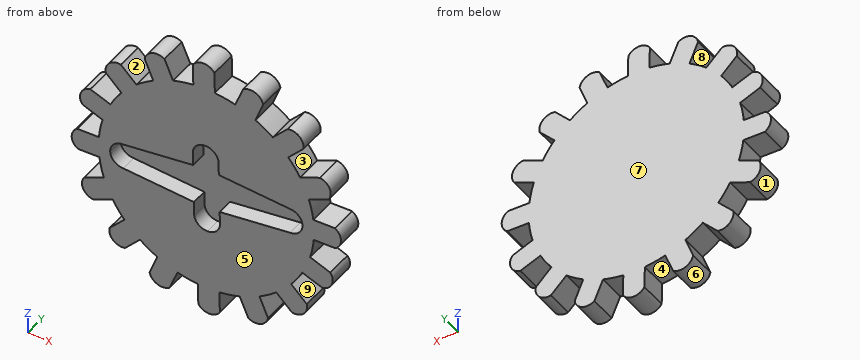
```python
from build123d import *

# Parameters (mm, degrees)
EXTRUDE001_DEPTH                      = 3
EXTRUDE001_ONTO_SKETCH001_ROLL_ANGLE  = -90
EXTRUDE001_ONTO_SKETCH001_PITCH_ANGLE = -1.786809
EXTRUDE_DEPTH                         = 5
EXTRUDE_ONTO_SKETCH_ROLL_ANGLE        = -90
EXTRUDE_ONTO_SKETCH_PITCH_ANGLE       = -1.786809
CUT_PITCH_ANGLE                       = 3
CUT_PLACEMENT_ANGLE                   = 180


with BuildPart() as servo_horn_gap:
    # Sketch001 as drawn → Extrude001 (new)
    with BuildSketch(Plane.XY):
        with BuildLine():
            Line((-2.39133, 6.362213), (-2.39133, 3.691866))
            Line((-2.39133, 3.691866), (-15.4752, 2.398726))
            ThreePointArc((-15.4752, 2.398726), (-17.158439, 1.689111), (-17.85396, 0))
            ThreePointArc((-17.85396, 0), (-17.158439, -1.689111), (-15.4752, -2.398726))
            Line((-2.39133, -3.691866), (-15.4752, -2.398726))
            Line((-2.39133, -6.362213), (-2.39133, -3.691866))
            ThreePointArc((-2.39133, -6.362213), (-1.613755, -7.907248), (0, -8.529784))
            ThreePointArc((0, -8.529784), (1.613755, -7.907248), (2.39133, -6.362213))
            Line((2.39133, -6.362213), (2.39133, -3.691866))
            Line((2.39133, -3.691866), (15.4752, -2.398726))
            ThreePointArc((15.4752, -2.398726), (17.158439, -1.689111), (17.85396, 0))
            ThreePointArc((17.85396, 0), (17.158439, 1.689111), (15.4752, 2.398726))
            Line((2.39133, 3.691866), (15.4752, 2.398726))
            Line((2.39133, 6.362213), (2.39133, 3.691866))
            ThreePointArc((2.39133, 6.362213), (1.613755, 7.907248), (0, 8.529784))
            ThreePointArc((0, 8.529784), (-1.613755, 7.907248), (-2.39133, 6.362213))
        make_face()
    extrude(amount=EXTRUDE001_DEPTH)


with BuildPart() as servo_horn_gap_1:
    # Extrude001 onto Sketch001 roll: moved
    add(servo_horn_gap.part.rotate(Axis((0, 0, 0), (1, 0, 0)), EXTRUDE001_ONTO_SKETCH001_ROLL_ANGLE))


with BuildPart() as servo_horn_gap_2:
    # Extrude001 onto Sketch001 pitch: moved
    add(servo_horn_gap_1.part.rotate(Axis((0, 0, 0), (0, 1, 0)), EXTRUDE001_ONTO_SKETCH001_PITCH_ANGLE))


with BuildPart() as servo_horn_gap_3:
    # Extrude001 onto Sketch001 placement: moved
    add(servo_horn_gap_2.part.moved(Location((16.5, 34.45, -6.25))))


with BuildPart() as servo_gear_mount:
    # Sketch as drawn → Extrude (new)
    with BuildSketch(Plane.XY):
        with BuildLine():
            ThreePointArc((-5.767545, -19.150337), (-3.901806, -19.615706), (-2, -19.899749))
            Line((-2, -19.899749), (-2, -23.899749))
            ThreePointArc((-2, -23.899749), (0, -25), (2, -23.899749))
            Line((2, -19.899749), (2, -23.899749))
            ThreePointArc((2, -19.899749), (3.901806, -19.615706), (5.767545, -19.150337))
            Line((5.767545, -19.150337), (7.298279, -22.845856))
            ThreePointArc((7.298279, -22.845856), (9.568651, -23.096339), (10.994375, -21.311783))
            Line((9.487389, -17.606518), (10.994375, -21.311783))
            ThreePointArc((9.487389, -17.606518), (11.122885, -16.621715), (12.657034, -15.485461))
            Line((12.657034, -15.485461), (15.485461, -18.313888))
            ThreePointArc((15.485461, -18.313888), (17.67767, -17.67767), (18.313888, -15.485461))
            Line((15.485461, -12.657034), (18.313888, -15.485461))
            ThreePointArc((15.485461, -12.657034), (16.621715, -11.122885), (17.606518, -9.487389))
            Line((17.606518, -9.487389), (21.311783, -10.994375))
            ThreePointArc((21.311783, -10.994375), (23.096339, -9.568651), (22.845856, -7.298279))
            Line((19.150337, -5.767545), (22.845856, -7.298279))
            ThreePointArc((19.150337, -5.767545), (19.615706, -3.901806), (19.899749, -2))
            Line((19.899749, -2), (23.899749, -2))
            ThreePointArc((23.899749, -2), (25, 0), (23.899749, 2))
            Line((19.899749, 2), (23.899749, 2))
            ThreePointArc((19.899749, 2), (19.615706, 3.901806), (19.150337, 5.767545))
            Line((19.150337, 5.767545), (22.845856, 7.298279))
            ThreePointArc((22.845856, 7.298279), (23.096339, 9.568651), (21.311783, 10.994375))
            Line((17.606518, 9.487389), (21.311783, 10.994375))
            ThreePointArc((17.606518, 9.487389), (16.621715, 11.122885), (15.485461, 12.657034))
            Line((15.485461, 12.657034), (18.313888, 15.485461))
            ThreePointArc((18.313888, 15.485461), (17.67767, 17.67767), (15.485461, 18.313888))
            Line((12.657034, 15.485461), (15.485461, 18.313888))
            ThreePointArc((12.657034, 15.485461), (11.122885, 16.621715), (9.487389, 17.606518))
            Line((9.487389, 17.606518), (10.994375, 21.311783))
            ThreePointArc((10.994375, 21.311783), (9.568651, 23.096339), (7.298279, 22.845856))
            Line((5.767545, 19.150337), (7.298279, 22.845856))
            ThreePointArc((5.767545, 19.150337), (3.901806, 19.615706), (2, 19.899749))
            Line((2, 19.899749), (2, 23.899749))
            ThreePointArc((2, 23.899749), (0, 25), (-2, 23.899749))
            Line((-2, 19.899749), (-2, 23.899749))
            ThreePointArc((-2, 19.899749), (-3.90256, 19.615556), (-5.769017, 19.149894))
            Line((-5.769017, 19.149894), (-7.300035, 22.845294))
            ThreePointArc((-7.300035, 22.845294), (-9.570426, 23.095604), (-10.996013, 21.310938))
            Line((-9.488742, 17.605788), (-10.996013, 21.310938))
            ThreePointArc((-9.488742, 17.605788), (-11.123524, 16.621288), (-12.657034, 15.485461))
            Line((-12.657034, 15.485461), (-15.485461, 18.313888))
            ThreePointArc((-15.485461, 18.313888), (-17.67767, 17.67767), (-18.313888, 15.485461))
            Line((-15.485461, 12.657034), (-18.313888, 15.485461))
            ThreePointArc((-15.485461, 12.657034), (-16.621288, 11.123524), (-17.605788, 9.488742))
            Line((-17.605788, 9.488742), (-21.310938, 10.996013))
            ThreePointArc((-21.310938, 10.996013), (-23.095604, 9.570426), (-22.845294, 7.300035))
            Line((-19.149894, 5.769017), (-22.845294, 7.300035))
            ThreePointArc((-19.149894, 5.769017), (-19.615556, 3.90256), (-19.899749, 2))
            Line((-19.899749, 2), (-23.899749, 2))
            ThreePointArc((-23.899749, 2), (-25, 0), (-23.899749, -2))
            Line((-19.899749, -2), (-23.899749, -2))
            ThreePointArc((-19.899749, -2), (-19.615556, -3.90256), (-19.149894, -5.769017))
            Line((-19.149894, -5.769017), (-22.845294, -7.300035))
            ThreePointArc((-22.845294, -7.300035), (-23.095604, -9.570426), (-21.310938, -10.996013))
            Line((-17.605788, -9.488742), (-21.310938, -10.996013))
            ThreePointArc((-17.605788, -9.488742), (-16.621333, -11.123457), (-15.485563, -12.656909))
            Line((-15.485563, -12.656909), (-18.314013, -15.485313))
            ThreePointArc((-18.314013, -15.485313), (-17.677812, -17.677527), (-15.485608, -18.313763))
            Line((-12.657158, -15.485359), (-15.485608, -18.313763))
            ThreePointArc((-12.657158, -15.485359), (-11.122952, -16.621671), (-9.487389, -17.606518))
            Line((-9.487389, -17.606518), (-10.994375, -21.311783))
            ThreePointArc((-10.994375, -21.311783), (-9.568651, -23.096339), (-7.298279, -22.845856))
            Line((-5.767545, -19.150337), (-7.298279, -22.845856))
        make_face()
    extrude(amount=EXTRUDE_DEPTH)


with BuildPart() as servo_gear_mount_1:
    # Extrude onto Sketch roll: moved
    add(servo_gear_mount.part.rotate(Axis((0, 0, 0), (1, 0, 0)), EXTRUDE_ONTO_SKETCH_ROLL_ANGLE))


with BuildPart() as servo_gear_mount_2:
    # Extrude onto Sketch pitch: moved
    add(servo_gear_mount_1.part.rotate(Axis((0, 0, 0), (0, 1, 0)), EXTRUDE_ONTO_SKETCH_PITCH_ANGLE))


with BuildPart() as servo_gear_mount_3:
    # Extrude onto Sketch placement: moved
    add(servo_gear_mount_2.part.moved(Location((16.5, 34.45, -6.25))))


with BuildPart() as servo_gear_mount_4:
    # Extrude placement: moved
    add(servo_gear_mount_3.part.moved(Location((0, -2, 0))))

    # Cut: cut Servo Horn Gap
    add(servo_horn_gap_3.part, mode=Mode.SUBTRACT)


with BuildPart() as servo_gear_mount_5:
    # Cut pitch: moved
    add(servo_gear_mount_4.part.rotate(Axis((0, 0, 0), (0, 1, 0)), CUT_PITCH_ANGLE))


with BuildPart() as servo_gear_mount_6:
    # Cut placement: moved
    add(servo_gear_mount_5.part.moved(Location((32.750343, 68.75, 0.986916))).rotate(Axis((32.750343, 68.75, 0.986916), (0, 0, 1)), CUT_PLACEMENT_ANGLE))


solid = servo_gear_mount_6.part
```
Verification items for the finished model (mm, model axes). Face numbers are marked on the shaded views. A direction names the side the tool comes from. Coordinates: 2 decimals unless noted, no trailing zeros. One line per item, written item: value.
Item 1: Access from +Z, -Z, +X, -X, +Y, -Y to the whole of each face (thin tool, end or side, straight path). Record for the marked faces 1, 2, 3, 4 and 5.
Check sheet entries:
face 1: -X, +Y, -Y
face 2: +Z, +Y, -Y
face 3: +Y, -Y
face 4: -Z, +Y, -Y
face 5: +Z, -Z, +X, -X, -Y
Item 2: Scan lines: line 1 along X through (y, z) = (33.35, -29); line 2 along X through (y, z) = (34.55, -28.5); line 3 along Z through (x, y) = (27.5, 32.95). Record each from-to range of solid material in increasing order.
Check sheet entries:
line 1: x = 6.84 to 9.83, 15.08 to 19.09, 24.74 to 26.67
line 2: x = 6.4 to 10.03, 15.07 to 19.07, 24.25 to 27.39
line 3: z = -28.38 to -25.93, -22.89 to -8.74, -3.04 to 10.65
Item 3: Mould release check, pull along Z, two halves, no side actions. Record for the marked faces 6, 7, 8 and 9: pulls with the +Z half, pulls with the -Z half, needs draft (parallel to the pull), parting line crosses it, or undercut.
Check sheet entries:
face 6: pulls with the -Z half
face 7: needs draft
face 8: undercut
face 9: undercut
Item 4: Gauge pin test, flat ends, axial feed: pin 1 Ø2 at (y, z) = (35, -8) entering from -X; pin 2 Ø3 at (y, z) = (35, 0.5) entering from +X. Record the tip position at first contact, or that the pin passes through.
Check sheet entries:
pin 1: stops at x = -8.36
pin 2: stops at x = 39.47
